Input: part model. Units: mm. Frame: model coordinates. A direction names the side the tool comes from. Coordinates: 2 decimals unless noted, no trailing zeros. Order: outer loops, then holes, each group sorted by start corner. A loop starts at its lowest first (then second) coordinate and runs counter-clockwise, first axis right, second up. Notation, with made-up numbers: (-6.75, -21) -> (15.25, -21) arc R37 cw to (15.25, 16) -> close; hole circle Ø1 at (-12.5, 75.5). An arc over 180 degrees is marked (long way). One line per item, written item: value. Start each with the question number.
from build123d import *

# Parameters (mm, degrees)
F0_W     = 1085
F0_H     = 938
F1_DEPTH = 70
F2_W     = 1120
F2_H     = 1000
F2_W_2   = 1085
F2_H_2   = 938
F3_DEPTH = 30
F4_W     = 309.3616962433
F4_H     = 93.0531620979
F5_DEPTH = 300
F6_R     = 40


with BuildPart() as f1:
    # F0 (on Front) → F1 (new body)
    with BuildSketch(Plane.XZ):
        Rectangle(F0_W, F0_H)
    extrude(amount=F1_DEPTH)

    # F2 (on face) → F3 (join)
    with BuildSketch(Plane.XZ.offset(70)):
        Rectangle(F2_W, F2_H)
        Rectangle(F2_W_2, F2_H_2, mode=Mode.SUBTRACT)
        Rectangle(F2_W_2, F2_H_2)
    extrude(amount=F3_DEPTH)

    # F4 (on face) → F5 (cut)
    with BuildSketch(Plane(origin=(0, 0, 0), x_dir=(-1, 0, 0), z_dir=(0, 1, 0))):
        with Locations((231.1289310455, 190.5976831913)):
            Rectangle(F4_W, F4_H)
    extrude(amount=-F5_DEPTH, mode=Mode.SUBTRACT)

    # F6
    f6_edges = [f1.edges().sort_by_distance(p)[0] for p in [
        (-560, -85, 500),
        (560, -85, 500),
        (560, -85, -500),
        (-560, -85, -500),
    ]]
    fillet(f6_edges, radius=F6_R)


solid = f1.part
1) Section query D-D, the plane x = 377. Return the cut outline in (y, z).
2) Access query for faces 1 (the cylindrical face through (-548.594, -85.21, 487.972)), 2 (the flat face through (-8, -35, -469)), 3 (the flat face through (-8, -35, 469)), 4 (the flat face through (542.5, -35, -7)), 5 (the flat face through (-385.81, -49, 190)). Directions: +Z, -Z, +X, -X, +Y, -Y. A direction counts if a zero-diameter tool reaches every point of the face in a straight line with its end or side. Return the directions, or none.
3) Section query A-A, the plane y = -20.5. Return the cut outline in (x, z).
4) Section query B-B, the plane x = -224. Return the cut outline in (y, z), plus the area to 3 significant figures.
5) Mould query, pull axis Z, two halves, no side actions, for faces 6 (the flat face through (-76.448, -49, 190)), 7 (the flat face through (-542.5, -35, -7)), 8 (the cylindrical face through (547.972, -85.21, -488.594)). Classes: +Z half, -Z half, draft (parallel to the pull), parting line (faces both ways), or undercut.
6) Pin query (flat end, axial travel): pin 1 Ø10 at (y, z) = (-44, 272) entering from +X; pin 2 Ø21 at (y, z) = (-29, 130.5) entering from -X; pin 3 Ø4 at (x, y) = (-430, -64.5) entering from -Z. Return the tip coordinate at first contact, or that it passes through.
7) Ray query, line 1 along X through (y, z) = (-40.5, 159); line 2 along Z through (x, y) = (-248, -86); line 3 along Z through (x, y) = (-258.5, -22). Return the intervals inside material, ascending. Write a range as from..to.
8) Section query C-C, the plane z = -255. Return the cut outline in (x, y).
Entries:
1. outline: (-100, -500) -> (-70, -500) -> (-70, -469) -> (0, -469) -> (0, 469) -> (-70, 469) -> (-70, 500) -> (-100, 500) -> close
2. face 1: +Z, -X, +Y, -Y
2. face 2: -Z, +X, -X, +Y
2. face 3: +Z, +X, -X, +Y
2. face 4: +Z, -Z, +X, +Y
2. face 5: +Y, -Y
3. outline: (-542.5, -469) -> (542.5, -469) -> (542.5, 469) -> (-542.5, 469) -> close; hole (-385.81, 144.07) -> (-76.45, 144.07) -> (-76.45, 237.12) -> (-385.81, 237.12) -> close
4. outline: (-100, -500) -> (-70, -500) -> (-70, -469) -> (0, -469) -> (0, 144.07) -> (-100, 144.07) -> close; (-100, 237.12) -> (0, 237.12) -> (0, 469) -> (-70, 469) -> (-70, 500) -> (-100, 500) -> close
4. area: 86,400 mm2
5. face 6: undercut
5. face 7: draft
5. face 8: -Z half
6. pin 1: stops at x = 542.5
6. pin 2: stops at x = -542.5
6. pin 3: stops at z = -469
7. line 1: x = -542.5..-385.81, -76.45..542.5
7. line 2: z = -500..144.07, 237.12..500
7. line 3: z = -469..144.07, 237.12..469
8. outline: (-560, -100) -> (560, -100) -> (560, -70) -> (542.5, -70) -> (542.5, 0) -> (-542.5, 0) -> (-542.5, -70) -> (-560, -70) -> close
